Here's how the part is built. I have some questions about the finished solid (model axes, mm). A direction names the side the tool comes from. Round coordinates to 2 decimals unless told otherwise and drop trailing zeros. Write each loop counter-clockwise with the first axis right and the second up, starting at its lowest first coordinate (ties: lowest second). Pieces come first, ordered by that corner, then holes. Notation, with made-up numbers: M -38.75,-3 L -10.75,-3 A17 ccw -10.75,18 Z; hole C 18.5,-34.5 d1. An arc over 180 degrees is marked long. Write item = value, one per line. Start each with the question number.
(1) On a 3-axis mill with a long thin cutter (end or side, diameter ignored), from which of +Z, -Z, +X, -X, +Y, -Y can I reach the whole of each face in a straight line? I mean faces 4 (the flat face through (49.5, -18, 26)), 5 (the flat face through (6, -5, 10)), 6 (the cylindrical face through (-4.287, -19.041, 16.794)). Say none if no direction works.
(2) I need wall thicknesses on line 1 along Z through (x, y) = (17, -2.05); line 2 along X through (y, z) = (-11, 29); line 3 along X through (y, z) = (-24, 29). Which ranges of each line are inside material? Lowest first, please.
(3) I want a section at A-A (z = 28.5). Give the number of separate pieces and of enclosed holes in the cut face, and give its area (3 significant figures).
(4) I want a section at B-B (y = -28). List the corners of the cut face in (x, z) for me.
(5) If we mould it in two halves opening along Z, with no side actions, what happens to faces 1 (the flat face through (2, -17, 15)), 2 (the cylindrical face through (28.29, -2.36, -17.27)), 3 (the flat face through (4.5, -22, 26))? For each: released by +Z, released by -Z, zero draft, split by the parting line, or undercut.
(6) Will these pins go through, and if not, where does the flat tip stop? pin 1 Ø13.5 at (y, z) = (-25, 20.5) entering from +X; pin 2 Ø13 at (x, y) = (3, -19.5) entering from -Z; pin 3 Ø4 at (x, z) = (5.5, -15) entering from -Y; pin 4 Ø0.6 at (y, z) = (-1.5, 5) entering from +X.
(7) I want a section at C-C (x = 17). List the corners of the cut face in (y, z) for me.
(8) I want a section at D-D (z = -14). List the corners of the cut face in (x, y) for me.
```python
from build123d import *

# Parameters (mm, degrees)
SALIENTE_EXTRUIR1_DEPTH  = 35
CROQUIS6_R               = 2.25
CROQUIS6_W               = 20
CROQUIS6_H               = 25
CORTAR_EXTRUIR3_DEPTH    = 10
CROQUIS7_R               = 2.25
SALIENTE_EXTRUIR4_DEPTH  = 15
CORTAR_EXTRUIR8_DEPTH    = 50
CORTAR_EXTRUIR11_REACH   = 69.158
CORTAR_EXTRUIR12_DEPTH   = 16
CROQUIS13_W              = 6.081292266
CROQUIS13_H              = 9.753773429
CORTAR_EXTRUIR13_DEPTH   = 15
CORTAR_EXTRUIR14_DEPTH   = 63.5
CORTAR_EXTRUIR15_DEPTH   = 100
SALIENTE_EXTRUIR5_REACH  = 69.158
CROQUIS16_W              = 15
CROQUIS16_H              = 10
CORTAR_EXTRUIR16_DEPTH   = 200
CORTAR_EXTRUIR17_DEPTH   = 200
SALIENTE_EXTRUIR7_DEPTH  = 23.5
CROQUIS22_R              = 2.25
CORTAR_EXTRUIR19_DEPTH   = 47
CORTAR_EXTRUIR20_DEPTH   = 31
CROQUIS24_W              = 29.420485752
CROQUIS24_H              = 5
SALIENTE_EXTRUIR9_DEPTH  = 10
CROQUIS25_R              = 1.75
CROQUIS25_R_2            = 1.5
CORTAR_EXTRUIR21_DEPTH   = 5
CROQUIS26_W              = 58.407198467
CROQUIS26_H              = 13.689988589
CORTAR_EXTRUIR22_DEPTH   = 73.871462178
CROQUIS27_W              = 5
CROQUIS27_H              = 10
SALIENTE_EXTRUIR10_DEPTH = 10
CORTAR_EXTRUIR23_START   = -10
CORTAR_EXTRUIR23_DEPTH   = 10


# Read off the part's stored shape, not the designer's step: Cortar-Extruir23
with BuildPart() as part:
    # Croquis1 → Saliente-Extruir1 (new body)
    with BuildSketch(Plane.XY):
        Polygon((0, 0), (45, 0), (52.5, -23), (40.5, -23), (40.5, -16.192411456), (32.5, -2), (12.5, -2), (4.5, -16), (4.5, -23), (-7.5, -23), align=None)
    extrude(amount=SALIENTE_EXTRUIR1_DEPTH)

    # Croquis6 → Cortar-Extruir3 (cut)
    with BuildSketch(Plane(origin=(0, 0, 0), x_dir=(1, 0, 0), z_dir=(0, 1, 0))):
        with Locations(Location((17, -28.5, 0), (0, 0, 180))):
            Circle(CROQUIS6_R)
        with Locations(Location((28, -28.5, 0), (0, 0, 270))):
            Circle(CROQUIS6_R)
        with Locations((22.5, -12.5)):
            Rectangle(CROQUIS6_W, CROQUIS6_H)
    extrude(amount=-CORTAR_EXTRUIR3_DEPTH, mode=Mode.SUBTRACT)

    # Cortar-Extruir11: up to this plane
    cortar_extruir11_end = Plane(origin=(50, -15, 0), z_dir=(0, -0.9079593845004518, -0.41905817746174695))
    # Croquis11 → Cortar-Extruir11 (cut, up to the surface)
    with BuildSketch(Plane.XZ.offset(23), mode=Mode.PRIVATE) as cortar_extruir11_sk1:
        with BuildLine():
            Line((-7.5, 15), (-7.5, -3.030649644))
            Line((-7.5, -3.030649644), (52.5, -3.030649644))
            Line((52.5, -3.030649644), (52.5, 15))
            ThreePointArc((52.5, 15), (22.5, 5.553378231), (-7.5, 15))
        make_face()
    cortar_extruir11_tool1 = split(extrude(cortar_extruir11_sk1.sketch, amount=-CORTAR_EXTRUIR11_REACH, mode=Mode.PRIVATE), bisect_by=cortar_extruir11_end, keep=Keep.BOTH, mode=Mode.PRIVATE)
    add(cortar_extruir11_tool1.solids().sort_by_distance((22.5, -23, 3.105508))[0], mode=Mode.SUBTRACT)

    # Croquis13 → Cortar-Extruir13 (cut)
    with BuildSketch(Plane.XY.offset(35)):
        with Locations((-7.540646133, -18.123113286)):
            Rectangle(CROQUIS13_W, CROQUIS13_H)
        with Locations((52.540646133, -18.123113286)):
            Rectangle(CROQUIS13_W, CROQUIS13_H)
    extrude(amount=-CORTAR_EXTRUIR13_DEPTH, mode=Mode.SUBTRACT)

    # Croquis14 → Cortar-Extruir14 (cut, symmetric)
    with BuildSketch(Plane(origin=(0, 0, 0), x_dir=(0, 0, -1), z_dir=(1, 0, 0))):
        Polygon((-15, -11), (-15, -28.858785619), (26, -23), (26, -3), align=None)
    extrude(amount=CORTAR_EXTRUIR14_DEPTH, both=True, mode=Mode.SUBTRACT)

    # Saliente-Extruir5: up to this face of the body (flat: up to its plane)
    saliente_extruir5_end = Plane(part.part.faces().sort_by_distance((6.25, 0, 0.570087713))[0])
    # Croquis16 → Saliente-Extruir5 (add, up to the picked face)
    with BuildSketch(Plane.XZ.offset(23), mode=Mode.PRIVATE) as saliente_extruir5_sk1:
        with Locations((5, 40)):
            Rectangle(CROQUIS16_W, CROQUIS16_H)
    saliente_extruir5_tool1 = split(extrude(saliente_extruir5_sk1.sketch, amount=-SALIENTE_EXTRUIR5_REACH, mode=Mode.PRIVATE), bisect_by=saliente_extruir5_end, keep=Keep.BOTH, mode=Mode.PRIVATE)
    # Croquis16 → Saliente-Extruir5 (add, up to the picked face)
    with BuildSketch(Plane.XZ.offset(23), mode=Mode.PRIVATE) as saliente_extruir5_sk2:
        with Locations((40, 40)):
            Rectangle(CROQUIS16_W, CROQUIS16_H)
    saliente_extruir5_tool2 = split(extrude(saliente_extruir5_sk2.sketch, amount=-SALIENTE_EXTRUIR5_REACH, mode=Mode.PRIVATE), bisect_by=saliente_extruir5_end, keep=Keep.BOTH, mode=Mode.PRIVATE)
    add(saliente_extruir5_tool1.solids().sort_by(Axis((5, -23, 40), (0, 1, 0)))[0])
    add(saliente_extruir5_tool2.solids().sort_by(Axis((40, -23, 40), (0, 1, 0)))[0])

    # Croquis17 → Cortar-Extruir16 (cut)
    with BuildSketch(Plane.ZY.offset(2.5)):
        Polygon((35, 0), (45, -23), (45, 0), align=None)
    extrude(amount=-CORTAR_EXTRUIR16_DEPTH, mode=Mode.SUBTRACT)

    # Croquis18 → Cortar-Extruir17 (cut)
    with BuildSketch(Plane(origin=(0, 0, 35), x_dir=(-1, 0, 0), z_dir=(0, 0, -1))):
        Polygon((-32.5, -2), (-40.5, -16.192411456), (-40.5, -23), (-32.5, -23), align=None)
        Polygon((-12.5, -23), (-4.5, -23), (-4.5, -16), (-12.5, -2), align=None)
        Polygon((-47.5, -7.666666667), (-45, 0), (-47.5, 0), align=None)
        Polygon((2.5, 0), (0, 0), (2.5, -7.666666667), align=None)
    extrude(amount=-CORTAR_EXTRUIR17_DEPTH, mode=Mode.SUBTRACT)



with BuildPart() as body_2:
    # Croquis7 → Saliente-Extruir4 (new body)
    with BuildSketch(Plane(origin=(0, 0, 0), x_dir=(1, 0, 0), z_dir=(0, 1, 0))):
        with BuildLine():
            Line((12.5, 16), (32.5, 16))
            Line((32.5, 16), (32.5, 0))
            Line((32.5, 0), (45, 0))
            Line((45, 0), (40.044296858, 18.577458823))
            ThreePointArc((40.044296858, 18.577458823), (36.474189304, 23.930150952), (30.382169451, 26))
            Line((30.382169451, 26), (14.617830549, 26))
            ThreePointArc((14.617830549, 26), (8.525810696, 23.930150952), (4.955703142, 18.577458823))
            Line((4.955703142, 18.577458823), (0, 0))
            Line((0, 0), (12.5, 0))
            Line((12.5, 0), (12.5, 16))
        make_face()
        with Locations((28, 19.5)):
            Circle(CROQUIS7_R, mode=Mode.SUBTRACT)
        with Locations((17, 19.5)):
            Circle(CROQUIS7_R, mode=Mode.SUBTRACT)
    extrude(amount=-SALIENTE_EXTRUIR4_DEPTH)

    # Croquis10 → Cortar-Extruir8 (cut)
    with BuildSketch(Plane(origin=(0, 0, 0), x_dir=(0, 0, -1), z_dir=(1, 0, 0))):
        Polygon((0, -15), (26, -3), (26, 0), (28.244981963, 0), (28.244981963, -21.856093693), align=None)
    extrude(amount=CORTAR_EXTRUIR8_DEPTH, mode=Mode.SUBTRACT)

    # Croquis12 → Cortar-Extruir12 (cut)
    with BuildSketch(Plane.XY):
        Polygon((12.5, -2), (12.5, -7.5), (12.5, -22.325980529), (0.885153984, -22.325980529), align=None)
        Polygon((44.114846016, -22.325980529), (32.5, -22.325980529), (32.5, -7.5), (32.5, -2), align=None)
    extrude(amount=-CORTAR_EXTRUIR12_DEPTH, mode=Mode.SUBTRACT)

    # Croquis15 → Cortar-Extruir15 (cut, symmetric)
    with BuildSketch(Plane(origin=(0, 0, 0), x_dir=(0, 0, -1), z_dir=(1, 0, 0))):
        Polygon((-15, -23), (-15, -11), (26, -3), align=None)
    extrude(amount=CORTAR_EXTRUIR15_DEPTH, both=True, mode=Mode.SUBTRACT)


with BuildPart() as part_1:
    add(part.part)

    add(body_2.part)  # Saliente-Extruir7 merges body 2
    # Croquis20 → Saliente-Extruir7 (add, symmetric)
    with BuildSketch(Plane(origin=(22.5, 0, 0), x_dir=(0, 0, -1), z_dir=(1, 0, 0))):
        Polygon((-15, -11), (-15, 0), (26, 0), (26, -3), align=None)
    extrude(amount=SALIENTE_EXTRUIR7_DEPTH, both=True)

    # Croquis22 → Cortar-Extruir19 (cut)
    with BuildSketch(Plane(origin=(0, 0, 0), x_dir=(1, 0, 0), z_dir=(0, 1, 0))):
        with Locations(Location((17, 19.5, 0), (0, 0, 180))):
            Circle(CROQUIS22_R)
        with Locations(Location((28, 19.5, 0), (0, 0, 180))):
            Circle(CROQUIS22_R)
        Polygon((12.5, 0), (12.5, -25), (32.5, -25), (32.5, 0), (32.5, 16), (12.5, 16), align=None)
        with BuildLine():
            Line((4.955703142, 18.577458823), (-2.632555673, 0))
            Line((-2.632555673, 0), (-11.688532454, 0))
            Line((-11.688532454, 0), (-11.688532454, 31.257495622))
            Line((-11.688532454, 31.257495622), (0, 31.257495622))
            Line((0, 31.257495622), (45, 31.257495622))
            Line((45, 31.257495622), (54.896993635, 31.257495622))
            Line((54.896993635, 31.257495622), (58.873924375, 0))
            Line((58.873924375, 0), (47.632555673, 0))
            Line((47.632555673, 0), (40.044296858, 18.577458823))
            ThreePointArc((40.044296858, 18.577458823), (36.474189304, 23.930150952), (30.382169451, 26))
            Line((30.382169451, 26), (14.617830549, 26))
            ThreePointArc((14.617830549, 26), (8.525810696, 23.930150952), (4.955703142, 18.577458823))
        make_face()
    extrude(amount=-CORTAR_EXTRUIR19_DEPTH, mode=Mode.SUBTRACT)

    # Croquis23 → Cortar-Extruir20 (cut)
    with BuildSketch(Plane.XY.offset(15)):
        Polygon((7.357142857, -11), (12.5, -11), (12.5, -2), align=None)
        Polygon((37.573133641, -11), (32.5, -2), (32.5, -11), align=None)
    extrude(amount=-CORTAR_EXTRUIR20_DEPTH, mode=Mode.SUBTRACT)

    # Croquis24 → Saliente-Extruir9 (add)
    with BuildSketch(Plane.XY.offset(35)):
        with Locations((22.884581513, -2.5)):
            Rectangle(CROQUIS24_W, CROQUIS24_H)
    extrude(amount=-SALIENTE_EXTRUIR9_DEPTH)

    # Croquis25 → Cortar-Extruir21 (cut)
    with BuildSketch(Plane(origin=(0, 0, 0), x_dir=(1, 0, 0), z_dir=(0, 1, 0))):
        with Locations(Location((17, -28.5, 0), (0, 0, 180))):
            Circle(CROQUIS25_R)
        with Locations((28, -28.5)):
            Circle(CROQUIS25_R)
        with Locations(Location((6.253029256, -10.000000184, 0), (0, 0, 180))):
            Circle(CROQUIS25_R_2)
        with Locations((38.746970744, -10.000000184)):
            Circle(CROQUIS25_R_2)
    extrude(amount=-CORTAR_EXTRUIR21_DEPTH, mode=Mode.SUBTRACT)

    # Croquis26 → Cortar-Extruir22 (cut, through all)
    with BuildSketch(Plane(origin=(0, 0, 0), x_dir=(1, 0, 0), z_dir=(0, 1, 0))):
        with Locations((24.703599234, -39.344994294)):
            Rectangle(CROQUIS26_W, CROQUIS26_H)
    extrude(amount=-CORTAR_EXTRUIR22_DEPTH, mode=Mode.SUBTRACT)

    # Croquis27 → Saliente-Extruir10 (add)
    with BuildSketch(Plane.XZ.offset(23)):
        with Locations((2, 27.5)):
            Rectangle(CROQUIS27_W, CROQUIS27_H)
        with Locations((42.976758833, 27.5)):
            Rectangle(CROQUIS27_W, CROQUIS27_H)
    extrude(amount=SALIENTE_EXTRUIR10_DEPTH)

    # Cortar-Extruir23 outline → Cortar-Extruir23 (cut)
    with BuildSketch(Plane.XZ.offset(23).offset(CORTAR_EXTRUIR23_START)):
        with BuildLine():
            ThreePointArc((-2.152586071, 15), (-4.921729811, 17.378723686), (-7.462476533, 20))
            Line((-7.462476533, 20), (-9, 21.738415502))
            Line((-9, 21.738415502), (-9, 15))
            Line((-9, 15), (-2.152586071, 15))
        make_face()
        with BuildLine():
            ThreePointArc((52.462476533, 20), (49.921729811, 17.378723686), (47.152586071, 15))
            Line((47.152586071, 15), (54, 15))
            Line((54, 15), (54, 21.738415502))
            Line((54, 21.738415502), (52.462476533, 20))
        make_face()
    extrude(amount=CORTAR_EXTRUIR23_DEPTH, mode=Mode.SUBTRACT)


solid = part_1.part
```
Returned:
q1.face_4 = +Z, +X, +Y, -Y
q1.face_5 = +Y
q1.face_6 = -Z, -X, -Y
q2.line_1 = -26 to -21.75, -17.25 to -16, 25 to 26.75, 30.25 to 32.5
q2.line_2 = -3.59 to 7.36, 37.57 to 48.59
q2.line_3 = -0.5 to 4.5, 40.48 to 45.48
q3.separate_pieces = 3
q3.enclosed_holes = 0
q3.area = 667 mm²
q4.outline = M -0.5,22.5 L 4.5,22.5 L 4.5,32.5 L -0.5,32.5 Z; M 40.48,22.5 L 45.48,22.5 L 45.48,32.5 L 40.48,32.5 Z
q5.face_1 = released by -Z
q5.face_2 = undercut
q5.face_3 = zero draft
q6.pin_1 = 52.46
q6.pin_2 = 15
q6.pin_3 = -5.54
q6.pin_4 = 46
q7.outline = M -5,25 L 0,25 L 0,26.75 L -5,26.75 Z; M -5,30.25 L 0,30.25 L 0,32.5 L -5,32.5 Z; M -4.95,-16 L -4.71,-17.25 L 0,-17.25 L 0,-16 Z; M -3.83,-21.75 L -3,-26 L 0,-26 L 0,-21.75 Z
q8.outline = M 3.09,-5.34 L 10.59,-5.34 L 12.5,-2 L 12.5,0 L 3.09,0 Z; M 32.5,-2 L 34.38,-5.34 L 41.91,-5.34 L 41.91,0 L 32.5,0 Z
